Model file for the job. Use its own axes, mm. Face numbers are marked on the shaded views. A direction names the side the tool comes from. Coordinates: 2 decimals unless noted, no trailing zeros. Loops run counter-clockwise (first coordinate to the right, second up) from the corner with the lowest first, then second, coordinate; pieces in that order, holes last.
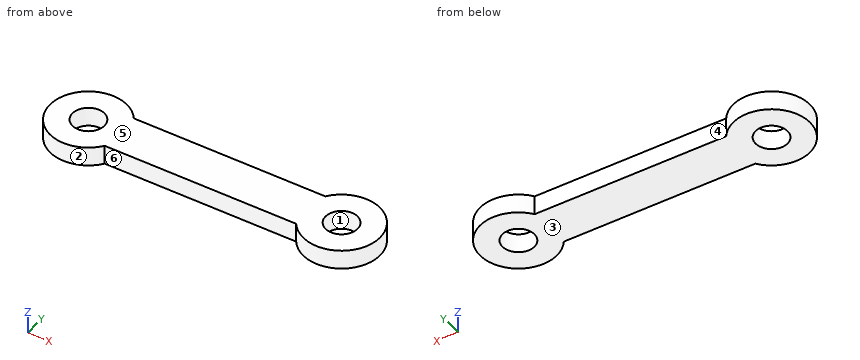
from build123d import *

# Parameters (mm, degrees)
EXTRUDE_START       = -3
EXTRUDE_1_DEPTH     = 6
SKETCH_2_R          = 5
CUT_EXTRUDE_1_DEPTH = 54.702886895


# Read off the part's stored shape, not the designer's step: 凸台-拉伸1
with BuildPart() as part:
    # 凸台-拉伸1 outline → 凸台-拉伸1 (new body)
    with BuildSketch(Plane.XY.offset(EXTRUDE_START)):
        with BuildLine():
            ThreePointArc((30.2532, -7), (52, 0), (30.2532, 7))
            Line((30.2532, 7), (-30.2532, 7))
            ThreePointArc((-30.2532, 7), (-52, 0), (-30.2532, -7))
            Line((-30.2532, -7), (30.2532, -7))
        make_face()
    extrude(amount=EXTRUDE_1_DEPTH)

    # 草图2 → 切除-拉伸1 (cut, through all)
    with BuildSketch(Plane.XY.offset(3)):
        with Locations((-40, 0)):
            Circle(SKETCH_2_R)
        with Locations((40, 0)):
            Circle(SKETCH_2_R)
    extrude(amount=-CUT_EXTRUDE_1_DEPTH, mode=Mode.SUBTRACT)


solid = part.part
Q1. Which spindle directions (+Z, -Z, +X, -X, +Y, -Y) get a long thin tool onto all of the face, cutting with end or side? Do the marked faces 4, 5 and 6. Say none if no direction does.
Answers:
face 4: +Z, -Z, +Y
face 5: +Z, +X, -X, +Y, -Y
face 6: +Z, -Z, -Y
Q2. Flat gauge pins, fed straight in: P1, Ø1.8, axis at x = 3.5, z = 0.5, coming from the +Y side; P2, Ø1, axis at y = -6, z = 1, coming from the -X side; P3, Ø1.5, axis at x = 8.5, z = 2, coming from the -Y side. Where does each tip first touch, or does it go through?
Answers:
P1: stops at y = 7
P2: stops at x = -50.67
P3: stops at y = -7
Q3. Mould opens along Y. For the marked faces 1, 2 and 3 say: +Y half, -Y half, draft (parallel to the pull), parting line (faces both ways), or undercut.
Answers:
face 1: undercut
face 2: parting line
face 3: draft
Q4. Slice it at A-A (y = 0). List the corners of the cut face in (x, z).
Answers:
outline: (-52, -3) - (-45, -3) - (-45, 3) - (-52, 3) - close; (-35, -3) - (35, -3) - (35, 3) - (-35, 3) - close; (45, -3) - (52, -3) - (52, 3) - (45, 3) - close
Q5. Slice it at B-B (x = 40). List the corners of the cut face in (y, z), and give its area (3 significant figures).
Answers:
outline: (-12, -3) - (-5, -3) - (-5, 3) - (-12, 3) - close; (5, -3) - (12, -3) - (12, 3) - (5, 3) - close
area: 84.0 mm2
Q6. Slice it at C-C (z = -1.7). List the corners of the cut face in (x, y).
Answers:
outline: (-30.25, -7) - (30.25, -7) arc R12 ccw (long way) to (30.25, 7) - (-30.25, 7) arc R12 ccw (long way) to start; hole circle Ø10 at (-40, 0); hole circle Ø10 at (40, 0)
Q7. Slice it at D-D (x = -18.5). List the corners of the cut face in (y, z), and give its area (3 significant figures).
Answers:
outline: (-7, -3) - (7, -3) - (7, 3) - (-7, 3) - close
area: 84.0 mm2
Q8. Drill centre lines: line 1 (Y direction, x = -40, z = -0.7); line 2 (X direction, y = 0.5, z = -2.5); line 3 (X direction, y = 3.5, z = 2.25). Where is each one in solid material? Low to high.
Answers:
line 1: y = -12 to -5, 5 to 12
line 2: x = -51.99 to -44.97, -35.03 to 35.03, 44.97 to 51.99
line 3: x = -51.48 to -43.57, -36.43 to 36.43, 43.57 to 51.48
